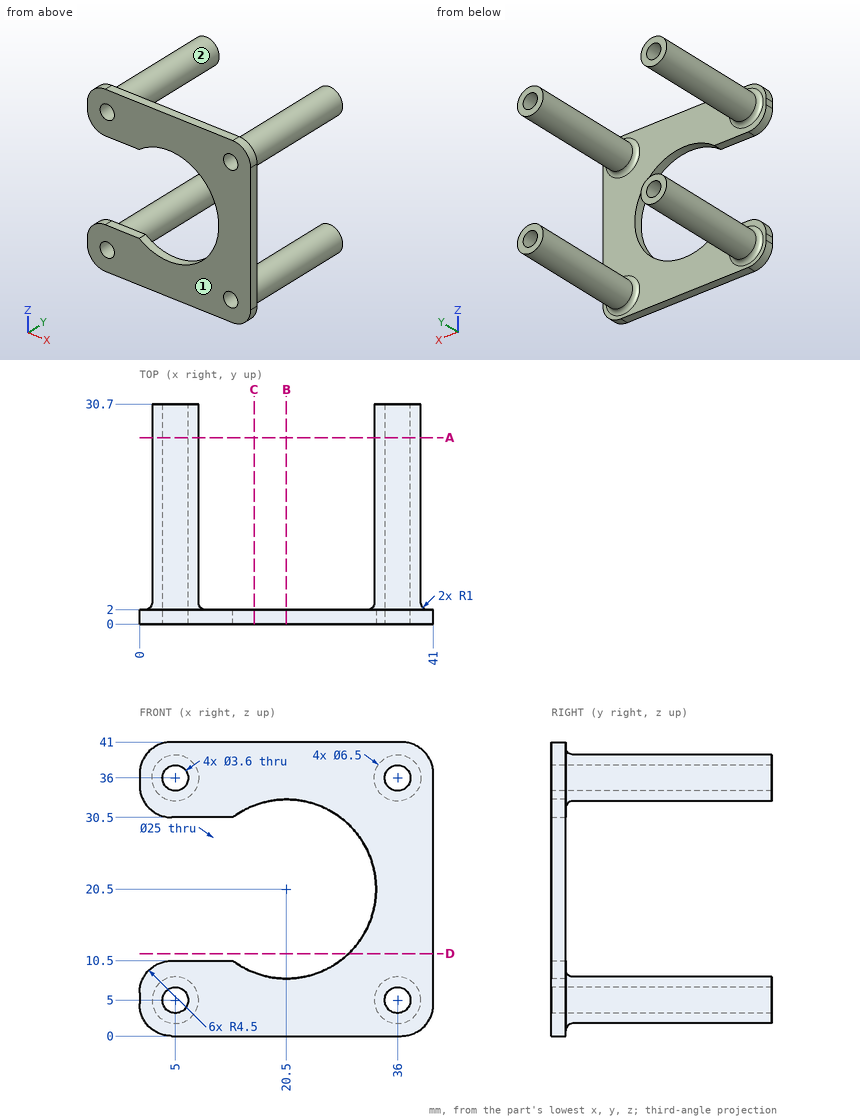
Design review of the part shown in the three views and the two pictorial views. Dimensions are in mm from the part's minimum x, y and z. Coordinates: 2 decimals unless noted, no trailing zeros. Write each loop counter-clockwise with the first axis right and the second up, starting at its lowest first coordinate (ties: lowest second). Pieces come first, ordered by that corner, then holes.
(1) Add section C-C on x = 16. Give the boundary of the cut face in (y, z), then the cut area to 3 significant figures.
(2) Add section B-B on x = 20.5. Give the boundary of the cut face in (y, z).
(3) Add section A-A on y = 26. Give the boundary of the cut face in (x, z).
(4) The part is to be moulded in two halves that separate along Z. For the marked faces 1 and 2, say which applies: +Z half, -Z half, draft (parallel to the pull), parting line (faces both ways), or undercut.
(5) Add section D-D on z = 11.5. Give the boundary of the cut face in (x, y).
(6) Wall thickness on probe 1 along X at (y, z) = (20, 5); probe 2 along Z at (x, y) = (20, 1): over which ranges is each line inside the solid? List them lowest first.
(7) For pin 1 Ø6 at (y, z) = (12, 32.5) entering from -X; pin 2 Ø2 at (x, z) = (5, 36) entering from -Y; pin 3 Ø4.5 at (x, z) = (5, 5) entering from -Y; pin 4 Ø8 at (x, y) = (32.5, 20.5) entering from +Z, all flat-tipped, find the tip position at first contact; note any pin that passes through.
Answer sheet:
1. outline: (0, 0) - (2, 0) - (2, 8.84) - (0, 8.84) - close; (0, 32.16) - (2, 32.16) - (2, 41) - (0, 41) - close
1. area: 35.4 mm2
2. outline: (0, 0) - (2, 0) - (2, 8) - (0, 8) - close; (0, 33) - (2, 33) - (2, 41) - (0, 41) - close
3. outline: circle Ø6.5 at (5, 5); circle Ø6.5 at (5, 36); circle Ø6.5 at (36, 5); circle Ø6.5 at (36, 36); hole circle Ø3.6 at (5, 5); hole circle Ø3.6 at (5, 36); hole circle Ø3.6 at (36, 5); hole circle Ø3.6 at (36, 36)
4. face 1: draft
4. face 2: undercut
5. outline: (29.17, 0) - (41, 0) - (41, 2) - (29.17, 2) - close
6. probe 1: x = 1.75 to 3.2, 6.8 to 8.25, 32.75 to 34.2, 37.8 to 39.25
6. probe 2: z = 0 to 8.01, 32.99 to 41
7. pin 1: stops at x = 1.79
7. pin 2: passes through
7. pin 3: stops at y = 0
7. pin 4: stops at z = 39.25
